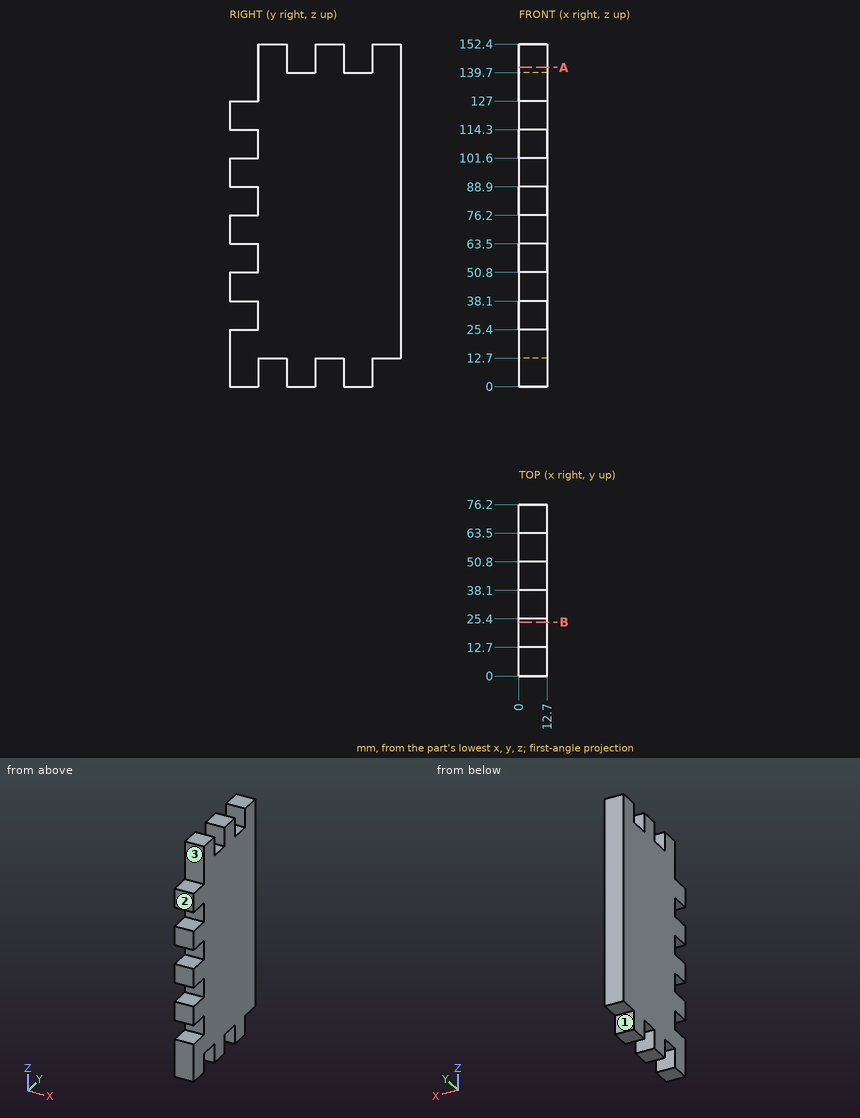
Could you check a few things on this drawing? It's one solid part, dimensions in mm from its lowest x, y, z. A direction names the side the tool comes from. Round coordinates to 2 decimals unless told otherwise and drop trailing zeros. Loops run counter-clockwise (first coordinate to the right, second up) from the corner with the lowest first, then second, coordinate; pieces in that order, holes last. Notation, with made-up numbers: (9, 4) -> (43, 4) arc R12 cw to (43, 12) -> close; hole circle Ø9 at (2, 9). An arc over 180 degrees is marked (long way). Write each question's results on one line, items separated by ' | '.
(1) If I drill on L1, parallel to Z at x = 3.75, y = 9; L2, parallel to Y at x = 10.5, z = 88.5; L3, parallel to Z at x = 10.5, y = 52, over which ranges is the centre line in solid material (lowest first)?
Worked answers:
L1: 0 to 25.4, 38.1 to 50.8, 63.5 to 76.2, 88.9 to 101.6, 114.3 to 127 | L2: 12.7 to 76.2 | L3: 0 to 139.7
(2) For the marked faces 1, 2 and 3, which set-ups out of +Z, -Z, +X, -X, +Y, -Y let a thin tool reach every point of the face, with its end or its side?
Worked answers:
face 1: -Z, +X, -X, +Y | face 2: +Z, -Z, +X, -X, -Y | face 3: +Z, +X, -X, -Y
(3) If we section it at B-B, the plane y = 24: List the corners of the cut face in (x, z) for me.
Worked answers:
outline: (0, 12.7) -> (12.7, 12.7) -> (12.7, 152.4) -> (0, 152.4) -> close
(4) If we section it at A-A, the plane z = 142: List the corners of the cut face in (x, y) for me.
Worked answers:
outline: (0, 12.7) -> (12.7, 12.7) -> (12.7, 25.4) -> (0, 25.4) -> close; (0, 38.1) -> (12.7, 38.1) -> (12.7, 50.8) -> (0, 50.8) -> close; (0, 63.5) -> (12.7, 63.5) -> (12.7, 76.2) -> (0, 76.2) -> close
(5) For P1, Ø2, axis at x = 7.5, z = 118, coming from the -Y side; P2, Ø4, axis at x = 4.5, y = 20, coming from the -Z side; P3, Ø6.5, axis at x = 7, z = 4, coming from the +Y side; P4, Ø6, axis at x = 5, z = 106, coming from the -Y side, each with a flat end and sliding along its axis, tell me the tip position at first contact or that it passes through.
Worked answers:
P1: y = 0 | P2: z = 12.7 | P3: y = 63.5 | P4: y = 12.7
